Answer from the drawing. Dimensions are ordinates in mm from the lowest x, y and z of the part. A direction names the side the tool comes from. Coordinates: 2 decimals unless noted, no trailing zeros. Write each loop counter-clockwise with the first axis right and the second up, starting at its lowest first coordinate (ties: lowest second). Pieces come first, ordered by that corner, then holes.
(1) The part is cut by section A-A on z = 4.75. Determine the outline of the cut face in (x, y).
(2) Straight lines are drawn through the part: line 1 (Z direction, x = 5.5, y = 6); line 2 (Z direction, x = 2, y = 5.75); line 3 (Y direction, x = 3.25, z = 2.5) (1 decimal). For each, find the intervals that lie inside material, in ascending order.
(3) For a pull along Z with two mould halves and no side action, classify the marked faces 1, 2 and 3 as +Z half, -Z half, draft (parallel to the pull), parting line (faces both ways), or undercut.
(4) The part is cut by section B-B on z = 3.75. Determine the outline of the cut face in (x, y).
(5) Given P1, Ø1, axis at x = 1.5, y = 1, coming from the +Z side; P2, Ø1.5, axis at x = 7, z = 6.5, coming from the +Y side (1 decimal); P3, Ø3, axis at y = 2, z = 3, coming from the -X side, each flat-ended and moving along its own axis, determine where each tip first touches the part or whether it passes through.
(6) Which of the six approach directions +Z, -Z, +X, -X, +Y, -Y give full straight-line access (tool end or side, diameter ignored) to the marked faces 4, 5 and 6?
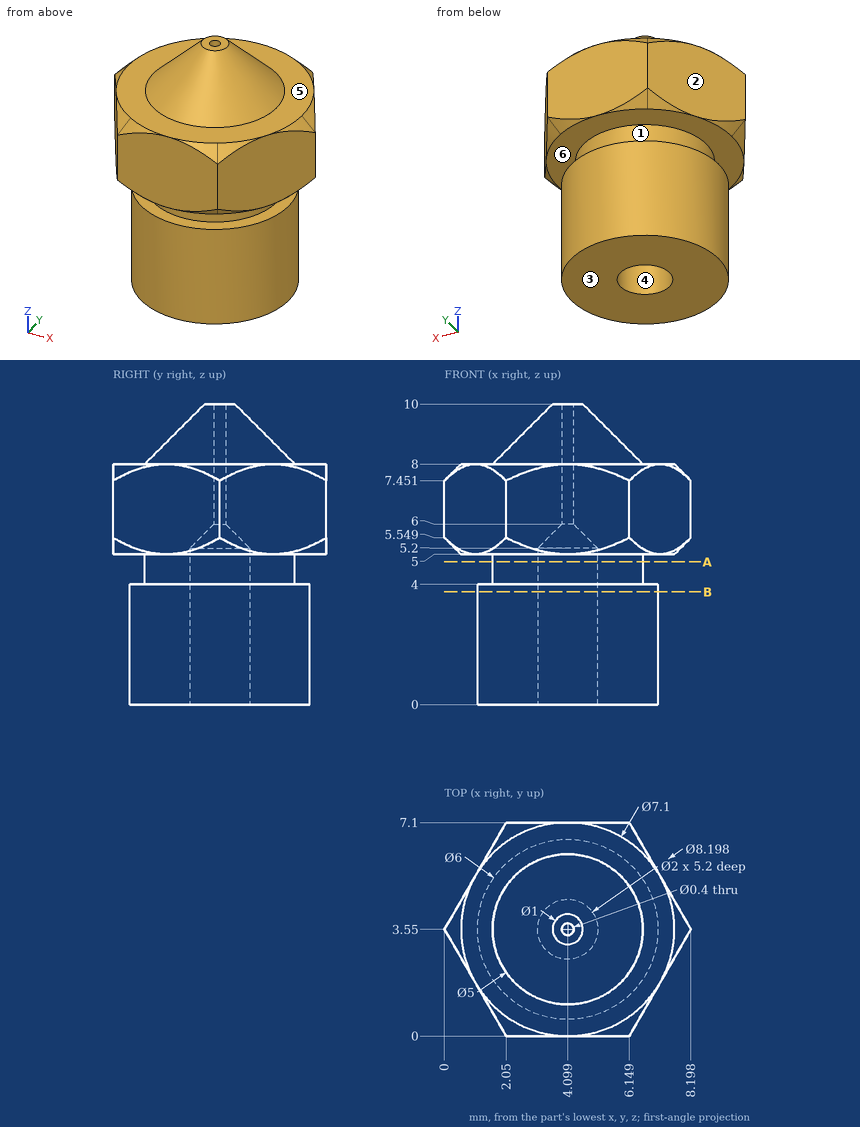
Model answer:
1. outline: circle Ø5 at (4.1, 3.55); hole circle Ø2 at (4.1, 3.55)
2. line 1: z = 0 to 4, 5 to 8
2. line 2: z = 5 to 8
2. line 3: y = 0.7 to 3, 4.1 to 6.4
3. face 1: undercut
3. face 2: draft
3. face 3: -Z half
4. outline: circle Ø6 at (4.1, 3.55); hole circle Ø2 at (4.1, 3.55)
5. P1: stops at z = 8
5. P2: stops at y = 6.9
5. P3: stops at x = 1.1
6. face 4: -Z
6. face 5: +Z
6. face 6: none
